Drawing for the job (mm, zero at the part's lowest x, y, z). Coordinates: 2 decimals unless noted, no trailing zeros. Write each loop counter-clockwise with the first axis right and the second up, starting at its lowest first coordinate (ties: lowest second). Pieces come first, ordered by that corner, then holes. Notation, with made-up numbers: (-37, 24) -> (16, 24) arc R12 cw to (16, 42) -> close; hole circle Ø9 at (-21.75, -2.75). An arc over 180 degrees is marked (long way). Answer as CSV lines item,"result". Start each with the question number.
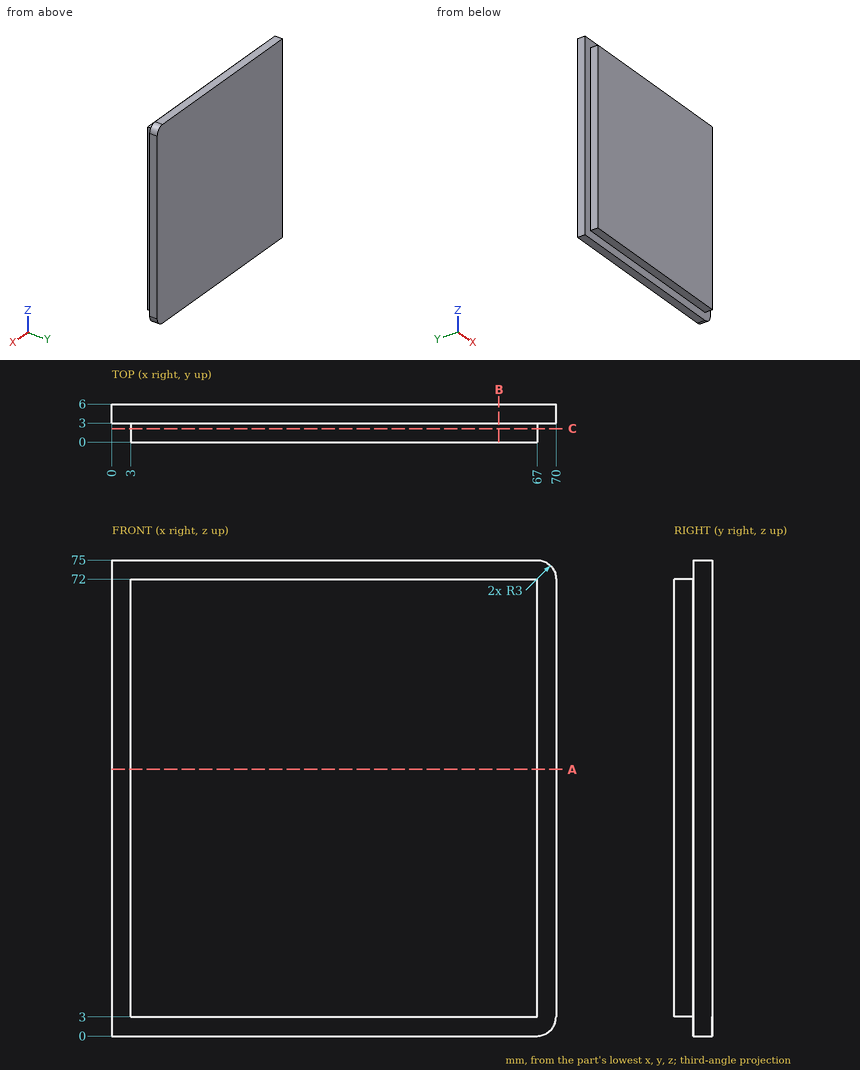
1. Cut at B-B (x = 61). Give the cut face in (y, z), then the cut area to 3 significant figures.
2. Flat gauge pins, fed straight in: P1, Ø0.9, axis at y = 2, z = 48.5, coming from the -X side; P2, Ø3.5, axis at y = 1, z = 53, coming from the +X side. Where does each tip first touch, or does it go through?
3. Cut at C-C (y = 2.1). Give the cut face in (x, z).
4. Cut at A-A (z = 42). Give the cut face in (x, y).
5. Wall check: line 1 (X direction, y = 1, z = 57); line 2 (Z direction, x = 24.5, y = 1.95). Give the ranges that are in metal, low to high.
Geometry check:
1,outline,"(0, 3) -> (3, 3) -> (3, 0) -> (6, 0) -> (6, 75) -> (3, 75) -> (3, 72) -> (0, 72) -> close"
1,area,"432 mm²"
2,P1,"x = 3"
2,P2,"x = 67"
3,outline,"(3, 3) -> (67, 3) -> (67, 72) -> (3, 72) -> close"
4,outline,"(0, 3) -> (3, 3) -> (3, 0) -> (67, 0) -> (67, 3) -> (70, 3) -> (70, 6) -> (0, 6) -> close"
5,line 1,"3 to 67"
5,line 2,"3 to 72"
